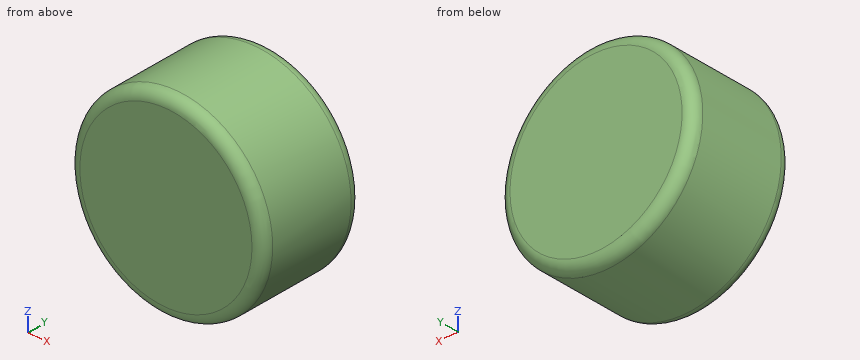
```python
from build123d import *

# Parameters (mm, degrees)
SKETCH_1_R          = 44.5
EXTRUDE_1_DEPTH     = 25
FILLET_1_R          = 5
SKETCH_9_R          = 40.5
CUT_EXTRUDE_1_DEPTH = 20.05


with BuildPart() as part:
    # 草图1 → 凸台-拉伸1 (new body, symmetric)
    with BuildSketch(Plane(origin=(0, 0, 0), x_dir=(1, 0, 0), z_dir=(0, 1, 0))):
        Circle(SKETCH_1_R)
    extrude(amount=EXTRUDE_1_DEPTH, both=True)

    # 圆角1
    fillet_1_edges = [part.edges().sort_by_distance(p)[0] for p in [
        (-44.5, -25, 0),
        (-44.5, 25, 0),
    ]]
    fillet(fillet_1_edges, radius=FILLET_1_R)

    # 草图9 → 切除-拉伸1 (cut, symmetric)
    with BuildSketch(Plane(origin=(0, 0, 0), x_dir=(1, 0, 0), z_dir=(0, 1, 0))):
        Circle(SKETCH_9_R)
    extrude(amount=CUT_EXTRUDE_1_DEPTH, both=True, mode=Mode.SUBTRACT)


solid = part.part
```
Work out the finished part from the listing and answer in its coordinate system (mm). Round coordinates to 2 decimals unless told otherwise and drop trailing zeros. Write each loop counter-clockwise with the first axis right and the second up, starting at its lowest first coordinate (ties: lowest second). Pieces come first, ordered by that corner, then holes.
1) Flat-ended cylindrical pins translate along their axes: P1, Ø4, axis at y = 14, z = 35, coming from the +X side; P2, Ø3, axis at y = 8, z = -6, coming from the +X side; P3, Ø6, axis at x = 16.5, y = -10.5, coming from the +Z side. Find the tip coordinate at first contact, or state that the pin passes through.
2) Consider probe 1 along Y at (x, z) = (3.5, 35); probe 2 along X at (y, z) = (10, 0). Determine where each line is inside the solid, lowest interval first.
3) A cutting plane is placed at C-C on y = 3.5. Determine the outline of the cut face in (x, z).
4) A cutting plane is placed at B-B on x = 0. Determine the outline of the cut face in (y, z).
5) A cutting plane is placed at A-A on z = 0. Determine the outline of the cut face in (x, y), and give its area (3 significant figures).
Entries:
1. P1: stops at x = 29.85
1. P2: stops at x = 44.27
1. P3: stops at z = 42.4
2. probe 1: y = -25 to -20.05, 20.05 to 25
2. probe 2: x = -44.5 to -40.5, 40.5 to 44.5
3. outline: circle Ø89 at (0, 0); hole circle Ø81 at (0, 0)
4. outline: (-25, -39.5) arc R5 ccw to (-20, -44.5) - (20, -44.5) arc R5 ccw to (25, -39.5) - (25, 39.5) arc R5 ccw to (20, 44.5) - (-20, 44.5) arc R5 ccw to (-25, 39.5) - close; hole (-20.05, -40.5) - (20.05, -40.5) - (20.05, 40.5) - (-20.05, 40.5) - close
5. outline: (-44.5, -20) arc R5 ccw to (-39.5, -25) - (39.5, -25) arc R5 ccw to (44.5, -20) - (44.5, 20) arc R5 ccw to (39.5, 25) - (-39.5, 25) arc R5 ccw to (-44.5, 20) - close; hole (-40.5, -20.05) - (40.5, -20.05) - (40.5, 20.05) - (-40.5, 20.05) - close
5. area: 1,180 mm2
